Read the model definition and answer for the solid it produces. Units are mm, in the model's axes. Face numbers are marked on the shaded views. Coordinates: 2 decimals unless noted, no trailing zeros. Loops run counter-clockwise (first coordinate to the right, second up) from the corner with the lowest first, then second, coordinate; pieces in that order, holes last. Notation, with made-up numbers: (25.25, 54) -> (45.25, 54) arc R11 cw to (45.25, 73) -> close; hole circle Ø1 at (82.25, -7.75). An arc over 180 degrees is marked (long way). Answer as a JSON object with one key per item and string values. Group by question number.
1) Determine the mould class of the marked faces 1, 2, 3 and 4 for opening direction X: released by +X, released by -X, zero draft, split by the parting line, or undercut.
2) Consider probe 1 along Z at (x, y) = (-6.25, 1.5); probe 2 along Y at (x, z) = (0, -3.1); probe 3 along Y at (x, z) = (0, -0.85). Determine where each line is inside the solid, lowest interval first. Write a range as [from, to].
3) Section A-A, the plane x = 0 is taken. Give the vertices of the cut face in (y, z).
4) Section C-C, the plane y = 0 is taken. Count the separate pieces of the cut face and the enclosed holes in it, plus the area to 3 significant figures.
5) Section B-B, the plane z = 2 is taken. Give the vertices of the cut face in (x, y), plus the area to 3 significant figures.
6) Flat-ended cylindrical pins translate along their axes: P1, Ø1.6, axis at y = 0.5, z = 1.5, coming from the -X side; P2, Ø0.7, axis at x = -10, y = 0, coming from the -Z side; P3, Ø1.1, axis at x = -10, y = 1, coming from the +Z side; P4, Ø4.5, axis at x = 0, y = 0, coming from the -Z side. Find the tip coordinate at first contact, or state that the pin passes through.
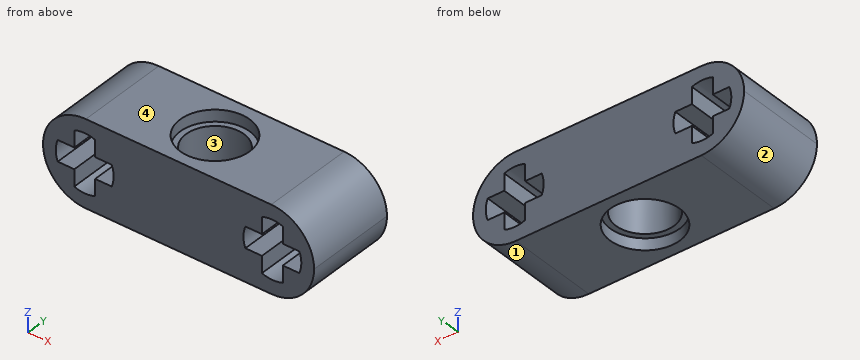
from build123d import *

# Parameters (mm, degrees)
F0_W     = 23.4
F0_H     = 7.4
F1_DEPTH = 3.95
F2_R     = 3.69999
F3_R     = 2.499
F4_DEPTH = 25
F3_R_2   = 3
F5_DEPTH = 1
F6_R     = 3
F6_R_2   = 2.499
F7_DEPTH = 1


# Not quite as in the source:
# - a fillet or chamfer is up to 0.001 mm smaller than in the source, because OpenCascade refuses the exact size


with BuildPart() as f1:
    # F0 (on Front) → F1 (new body, symmetric)
    with BuildSketch(Plane.XZ):
        Rectangle(F0_W, F0_H)
        with BuildLine():
            ThreePointArc((-7.199, -2.3313088598), (-8.099, -2.499), (-8.999, -2.3313088598))
            Line((-8.999, -2.3313088598), (-8.999, -0.9))
            Line((-8.999, -0.9), (-10.4303088598, -0.9))
            ThreePointArc((-10.4303088598, -0.9), (-10.598, 0), (-10.4303088598, 0.9))
            Line((-10.4303088598, 0.9), (-8.999, 0.9))
            Line((-8.999, 0.9), (-8.999, 2.3313088598))
            ThreePointArc((-8.999, 2.3313088598), (-8.099, 2.499), (-7.199, 2.3313088598))
            Line((-7.199, 2.3313088598), (-7.199, 0.9))
            Line((-7.199, 0.9), (-5.7676911402, 0.9))
            ThreePointArc((-5.7676911402, 0.9), (-5.6, 0), (-5.7676911402, -0.9))
            Line((-5.7676911402, -0.9), (-7.199, -0.9))
            Line((-7.199, -0.9), (-7.199, -2.3313088598))
        make_face(mode=Mode.SUBTRACT)
        with BuildLine():
            Line((7.199, 0.9), (7.199, 2.3313088598))
            ThreePointArc((7.199, 2.3313088598), (8.099, 2.499), (8.999, 2.3313088598))
            Line((8.999, 2.3313088598), (8.999, 0.9))
            Line((8.999, 0.9), (10.4303088598, 0.9))
            ThreePointArc((10.4303088598, 0.9), (10.598, 0), (10.4303088598, -0.9))
            Line((10.4303088598, -0.9), (8.999, -0.9))
            Line((8.999, -0.9), (8.999, -2.3313088598))
            ThreePointArc((8.999, -2.3313088598), (8.099, -2.499), (7.199, -2.3313088598))
            Line((7.199, -2.3313088598), (7.199, -0.9))
            Line((7.199, -0.9), (5.7676911402, -0.9))
            ThreePointArc((5.7676911402, -0.9), (5.6, 0), (5.7676911402, 0.9))
            Line((5.7676911402, 0.9), (7.199, 0.9))
        make_face(mode=Mode.SUBTRACT)
    extrude(amount=F1_DEPTH, both=True)

    # F2 (radius 3.7 in the source; OpenCascade refuses exactly that, so slightly less here)
    f2_edges = [f1.edges().sort_by_distance(p)[0] for p in [
        (-11.7, 0, -3.7),
        (-11.7, 0, 3.7),
        (11.7, 0, 3.7),
        (11.7, 0, -3.7),
    ]]
    fillet(f2_edges, radius=F2_R)

    # F3 (on face) → F4 (cut)
    with BuildSketch(Plane.XY.offset(3.7)):
        Circle(F3_R)
    extrude(amount=-F4_DEPTH, mode=Mode.SUBTRACT)

    # F3 (on face) → F5 (cut)
    with BuildSketch(Plane.XY.offset(3.7)):
        Circle(F3_R_2)
        Circle(F3_R, mode=Mode.SUBTRACT)
    extrude(amount=-F5_DEPTH, mode=Mode.SUBTRACT)

    # F6 (on face) → F7 (cut)
    with BuildSketch(Plane(origin=(0, 0, -3.7), x_dir=(1, 0, 0), z_dir=(0, 0, -1))):
        Circle(F6_R)
        Circle(F6_R_2, mode=Mode.SUBTRACT)
    extrude(amount=-F7_DEPTH, mode=Mode.SUBTRACT)


solid = f1.part
Determined:
{
 "1": {"face 1": "released by +X", "face 2": "released by -X", "face 3": "undercut", "face 4": "zero draft"},
 "2": {"probe 1": "[-3.7, -0.9], [0.9, 3.7]", "probe 2": "[-3.95, -3], [3, 3.95]", "probe 3": "[-3.95, -2.5], [2.5, 3.95]"},
 "3": {"outline": "(-3.95, -3.7) -> (-3, -3.7) -> (-3, -2.7) -> (-2.5, -2.7) -> (-2.5, 2.7) -> (-3, 2.7) -> (-3, 3.7) -> (-3.95, 3.7) -> close; (2.5, -2.7) -> (3, -2.7) -> (3, -3.7) -> (3.95, -3.7) -> (3.95, 3.7) -> (3, 3.7) -> (3, 2.7) -> (2.5, 2.7) -> close"},
 "4": {"separate pieces": "2", "enclosed holes": "2", "area": "93.7 mm²"},
 "5": {"outline": "(-11.11, -3.95) -> (-9, -3.95) -> (-9, 3.95) -> (-11.11, 3.95) -> close; (-7.2, -3.95) -> (7.2, -3.95) -> (7.2, 3.95) -> (-7.2, 3.95) -> close; (9, -3.95) -> (11.11, -3.95) -> (11.11, 3.95) -> (9, 3.95) -> close; hole circle Ø5 at (0, 0)", "area": "128 mm²"},
 "6": {"P1": "x = -11.63", "P2": "z = -3.31", "P3": "z = 3.4", "P4": "through"}
}
